Autodesk Inventor part; units mm, degrees
ref_plane "YZ Plane" through (0, 0, 0) normal (1, 0, 0) x (0, 1, 0)
ref_plane "XZ Plane" through (0, 0, 0) normal (0, 1, 0) x (-1, 0, 0)
ref_plane "XY Plane" through (0, 0, 0) normal (0, 0, 1) x (1, 0, 0)
sketch "Sketch1" plane through (0, 0, 0) normal (1, 0, 0) x (0, 1, 0)
  line L0 (-76.2, 88.9) -> (-76.2, 88.9)
  line L1 (-50.8, 127) -> (50.8, 127)
  line L2 (50.8, -127) -> (-50.8, -127)
  line L3 (-76.2, -88.9) -> (-76.2, 88.9)
  arc A0 (88.9, 88.9) -> (50.8, 127) centre (50.8, 88.9) ccw
  line L4 (76.2, 88.9) -> (88.9, 88.9)
  arc A1 (-50.8, 127) -> (-88.9, 88.9) centre (-50.8, 88.9) ccw
  line L5 (-50.8, 88.9) -> (-88.9, 88.9)
  arc A2 (50.8, -127) -> (88.9, -88.9) centre (50.8, -88.9) ccw
  line L6 (76.2, -88.9) -> (88.9, -88.9)
  line L7 (76.2, 88.9) -> (76.2, -88.9)
  arc A3 (-88.9, -88.9) -> (-50.8, -127) centre (-50.8, -88.9) ccw
  line L8 (-76.2, -88.9) -> (-88.9, -88.9)
  point P0 (0, 0)
  point P1 (-76.2, 117.2981)
  point P2 (-76.2, -117.2981)
  dimension "d62" = 254
  dimension "d64" = 76.2
  dimension "d65" = 127
  dimension "d66" = 76.2
  dimension "d72" = 76.2
  dimension "d73" = 25.4
  dimension "d74" = 76.2
  dimension "d76" = 25.4
  dimension "d77" = 76.2
  dimension "d78" = 25.4
extrude "Extrusion1" add sketch "Sketch1" along normal blind 6.35
sketch "Sketch3" plane through (6.35, 0, 0) normal (1, 0, 0) x (0, 0, -1)
  line L0 (88.9, 76.2) -> (-88.9, 76.2)
  line L1 (127, -50.8) -> (127, 50.8)
  line L2 (-88.9, -76.2) -> (88.9, -76.2)
  point P0 (0, 0)
  point P1 (0, -63.5)
  point P2 (0, 63.5)
  point P3 (0, 63.5)
  point P4 (127, 76.2)
  point P5 (127, -76.2)
  point P6 (-127, -76.2)
  dimension "d68" = 12.7
  dimension "d69" = 127
  dimension "d70" = 127
  dimension "d71" = 12.7
hole "Hole2" at (6.35, -63.5, 0) direction (-1, 0, 0) diameter 6.35 end through all
hole "Hole3" at (6.35, 63.5, 0) direction (-1, 0, 0) diameter 6.35 end through all
sketch "Sketch4" plane through (6.35, 0, 0) normal (1, 0, 0) x (0, 0, -1)
  line L0 (-127, 50.8) -> (-127, -50.8)
  line L1 (-127, 50.8) -> (127, 50.8)
  line L2 (127, 50.8) -> (127, -50.8)
  line L3 (127, -50.8) -> (-127, -50.8)
  line L4 (-127, -50.8) -> (-127, 50.8)
  point P0 (0, 0)
  point P1 (-88.9, 88.9)
  dimension "d79" = 101.6
  dimension "d80" = 38.1
extrude "Extrusion2" add sketch "Sketch4" against normal blind 19.05
sketch "Sketch5" plane through (6.35, -50.8, -127) normal (0, 0, -1) x (-1, 0, 0)
  line L0 (6.35, 0) -> (6.35, -38.1)
  line L1 (6.35, 101.6) -> (0, 101.6)
  line L2 (0, 0) -> (0, 101.6)
  point P0 (6.35, 50.8)
properties part number "Frame" material "ABS Plastic"
The model under review builds one solid part; all positions refer to its coordinate system, in mm. A direction names the side the tool comes from. Round coordinates to 2 decimals unless told otherwise and drop trailing zeros. Order: outer loops, then holes, each group sorted by start corner. A loop starts at its lowest first (then second) coordinate and runs counter-clockwise, first axis right, second up. Notation, with made-up numbers: (-33, 78) -> (10, 78) arc R12 cw to (10, 100) -> close; hole circle Ø6 at (5.25, 67.25). An arc over 180 degrees is marked (long way). One line per item, written item: value. Start each with the question number.
Q1. Take a section at A-A (x = 3). Write out the cut boundary in (y, z) (3 decimals).
Q2. Take a section at C-C (y = 63.5). Write out the cut boundary in (x, z) (3 decimals), and give its area (3 significant figures).
Q3. Machinability: for faces 4 (the face through (-6, -50.8, -2)), 5 (the face through (3, -82, -88.9)), 6 (the face through (3.13, 77.44, 116.14)), 7 (the face through (0, 70, 2)), 8 (the face through (3, 82, -88.9)), which of the approach directions +Z, -Z, +X, -X, +Y, -Y give a long, thin tool a straight path to every point of the face, cutting with its end or side? Answer none if there is none.
Q4. Take a section at D-D (z = 27). Write out the cut boundary in (x, y).
Q5. Clearance check with flat-ended pins moving along their axes: pin 1 Ø5 at (x, y) = (4, -82.5) entering from -Z; pin 2 Ø7 at (x, z) = (2.5, -6) entering from -Y; pin 3 Ø1.9 at (x, y) = (3.5, -80) entering from +Z; pin 4 Ø5 at (y, z) = (63.5, 0) entering from -X. State where each tip first meets the part, or that it passes through.
Q6. Wall thickness on line 1 (Y direction, x = 2.5, z = 0) (3 decimals); line 2 (Y direction, x = 5.5, z = 28.5); line 3 (X direction, y = 67, z = 82): over which ranges is each line inside the solid? List them lowest first.
Q7. Mouldability with a two-part tool opening along Z and no side actions: class faces 1 (the face through (3.131, -66.177, -1.707)), 2 (the face through (0, -70, 2)), 3 (the face through (3.13, 78.04, -115.54)) as released by +Z, released by -Z, zero draft, split by the parting line, or undercut.
Q8. Take a section at B-B (z = 0). Write out the cut boundary in (x, y) (3 decimals).
Reported:
1. outline: (-88.9, -88.9) arc R38.1 ccw to (-50.8, -127) -> (50.8, -127) arc R38.1 ccw to (88.9, -88.9) -> (76.2, -88.9) -> (76.2, 88.9) -> (88.9, 88.9) arc R38.1 ccw to (50.8, 127) -> (-50.8, 127) arc R38.1 ccw to (-88.9, 88.9) -> (-76.2, 88.9) -> (-76.2, -88.9) -> close; hole circle Ø6.35 at (-63.5, 0); hole circle Ø6.35 at (63.5, 0)
2. outline: (0, -124.821) -> (6.35, -124.821) -> (6.35, -3.175) -> (0, -3.175) -> close; (0, 3.175) -> (6.35, 3.175) -> (6.35, 124.821) -> (0, 124.821) -> close
2. area: 1,540 mm2
3. face 4: +Z, -Z, -X, -Y
3. face 5: +X, -X, -Y
3. face 6: +Z, +X, -X, +Y
3. face 7: +Z, -Z, -X, +Y
3. face 8: +X, -X, +Y
4. outline: (-12.7, -50.8) -> (0, -50.8) -> (0, -76.2) -> (6.35, -76.2) -> (6.35, 76.2) -> (0, 76.2) -> (0, 50.8) -> (-12.7, 50.8) -> close
5. pin 1: stops at z = -113.37
5. pin 2: stops at y = -76.2
5. pin 3: stops at z = 114.46
5. pin 4: passes through
6. line 1: y = -76.2 to -66.675, -60.325 to 60.325, 66.675 to 76.2
6. line 2: y = -76.2 to 76.2
6. line 3: x = 0 to 6.35
7. face 1: undercut
7. face 2: zero draft
7. face 3: released by -Z
8. outline: (-12.7, -50.8) -> (0, -50.8) -> (0, -60.325) -> (6.35, -60.325) -> (6.35, 60.325) -> (0, 60.325) -> (0, 50.8) -> (-12.7, 50.8) -> close; (0, -76.2) -> (6.35, -76.2) -> (6.35, -66.675) -> (0, -66.675) -> close; (0, 66.675) -> (6.35, 66.675) -> (6.35, 76.2) -> (0, 76.2) -> close
